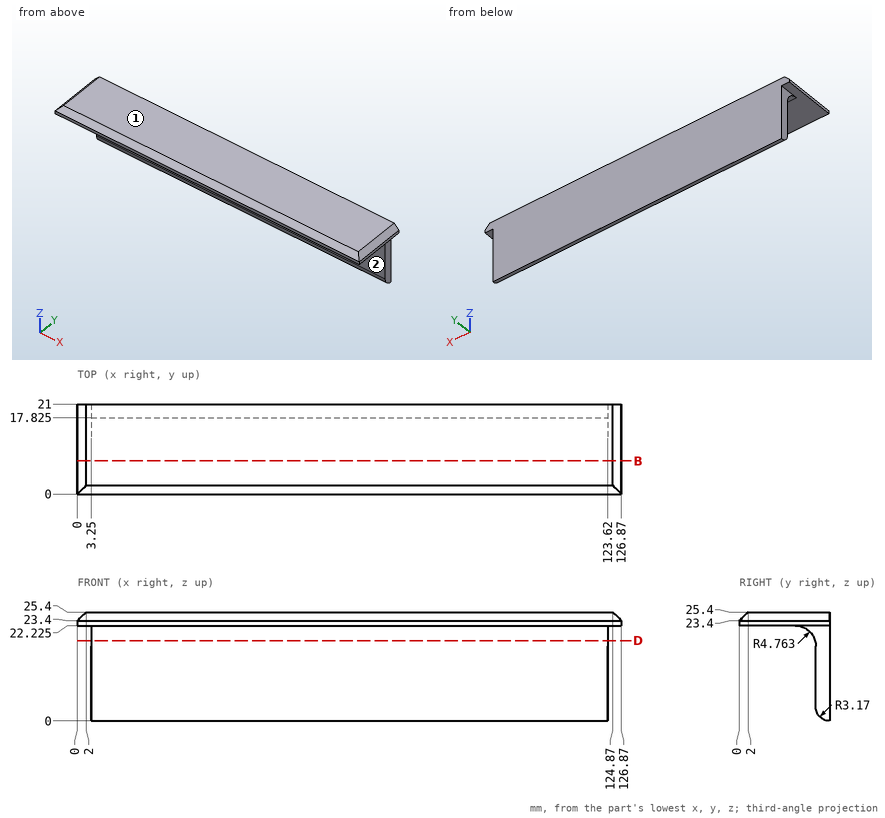
Drawing for the job (mm, zero at the part's lowest x, y, z). A direction names the side the tool comes from. Give positions to 0.01 mm unless a question says otherwise; leave off trailing zeros. Loops run counter-clockwise (first coordinate to the right, second up) from the corner with the lowest first, then second, coordinate; pieces in that order, holes last.
(1) Drill centre lines: line 1 along Y through (x, z) = (89.5, 3.75) (1 decimal); line 2 along X through (y, z) = (19, 11.75); line 3 along Z through (x, y) = (24, 5.25) (1 decimal). Where is each one in solid material? Low to high.
Return value:
line 1: y = 17.8 to 21
line 2: x = 3.25 to 123.62
line 3: z = 22.2 to 25.4
(2) Band-saw the part on B-B (y = 7.75). Write the cut outline in (x, z) (1 decimal), and give its area (3 significant figures).
Return value:
outline: (0, 22.2) - (126.9, 22.2) - (126.9, 23.4) - (124.9, 25.4) - (2, 25.4) - (0, 23.4) - close
area: 399 mm2
(3) Pin check, flat tips, straight feed: pin 1 (10 mm diameter, centred on y = 15.5, z = 10.5, fed in from -X); pin 2 (6.5 mm diameter, centred on y = 15.5, z = 12.5, fed in from +X); pin 3 (5 mm diameter, centred on x = 14, y = 5, fed in from -Z) (1 decimal). Stop position of each tip, or through.
Return value:
pin 1: stops at x = 3.25
pin 2: stops at x = 123.62
pin 3: stops at z = 22.2
(4) Band-saw the part on D-D (z = 18.75). Write the cut outline in (x, y).
Return value:
outline: (3.25, 17.65) - (123.62, 17.65) - (123.62, 21) - (3.25, 21) - close
(5) 3-axis set-ups, long thin cutter, end or side, ignore diameter. For the marked faces 1 and 2: which of +Z, -Z, +X, -X, +Y, -Y reach the whole face in a straight line?
Return value:
face 1: +Z, +X, -X, +Y, -Y
face 2: -Z, +X, -X, -Y
